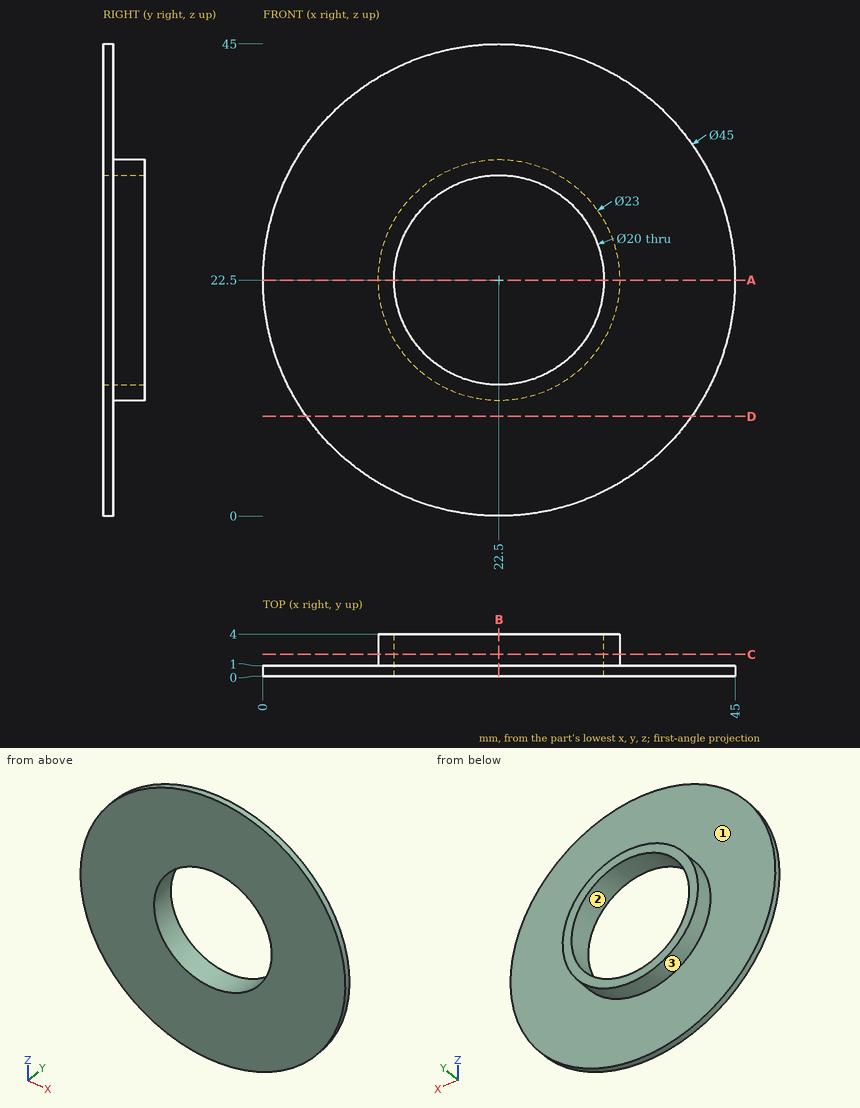
Print and shaded views of the part. All mm, measured from the part's lowest x, y and z. Round coordinates to 2 decimals unless told otherwise and drop trailing zeros. Write each loop counter-clockwise with the first axis right and the second up, starting at its lowest first coordinate (ties: lowest second). Pieces come first, ordered by that corner, then holes. Notation, with made-up numbers: (-35, 8) -> (1, 8) arc R21 cw to (1, 43) -> close; hole circle Ø2 at (27, -38.5). An arc over 180 degrees is marked (long way). Return JSON: item names as keys, results as strings. Group by question number.
Q1. Saw through at C-C on y = 2.05. Write the cut outline in (x, z).
Q2. Saw through at B-B on x = 22.5. Write the cut outline in (y, z).
Q3. Probe L1, parallel to X at y = 1.4, z = 22; L2, parallel to X at y = 0.9, z = 22.5; L3, parallel to Y at x = 34.5, z = 32.5. List the from-to ranges inside material, lowest first. Write a range as [from, to].
Q4. Pin check, flat tip, straight feed: pin 1 (4 mm diameter, centred on x = 6, z = 20.5, fed in from -Y). Stop position of the tip, or through.
Q5. Saw through at D-D on z = 9.5. Write the cut outline in (x, y), plus the area to 3 significant figures.
Q6. Saw through at A-A on z = 22.5. Write the cut outline in (x, y).
Q7. Mould opens along X. For the marked faces 1, 2 and 3 say: pulls with the +X half, pulls with the -X half, needs draft (parallel to the pull), parting line crosses it, or undercut.
Answer:
{
 "1": {"outline": "circle Ø23 at (22.5, 22.5); hole circle Ø20 at (22.5, 22.5)"},
 "2": {"outline": "(0, 0) -> (1, 0) -> (1, 11) -> (4, 11) -> (4, 12.5) -> (0, 12.5) -> close; (0, 32.5) -> (4, 32.5) -> (4, 34) -> (1, 34) -> (1, 45) -> (0, 45) -> close"},
 "3": {"L1": "[11.01, 12.51], [32.49, 33.99]", "L2": "[0, 12.5], [32.5, 45]", "L3": "[0, 1]"},
 "4": {"pin 1": "y = 0"},
 "5": {"outline": "(4.14, 0) -> (40.86, 0) -> (40.86, 1) -> (4.14, 1) -> close", "area": "36.7 mm2"},
 "6": {"outline": "(0, 0) -> (12.5, 0) -> (12.5, 4) -> (11, 4) -> (11, 1) -> (0, 1) -> close; (32.5, 0) -> (45, 0) -> (45, 1) -> (34, 1) -> (34, 4) -> (32.5, 4) -> close"},
 "7": {"face 1": "needs draft", "face 2": "undercut", "face 3": "parting line crosses it"}
}
